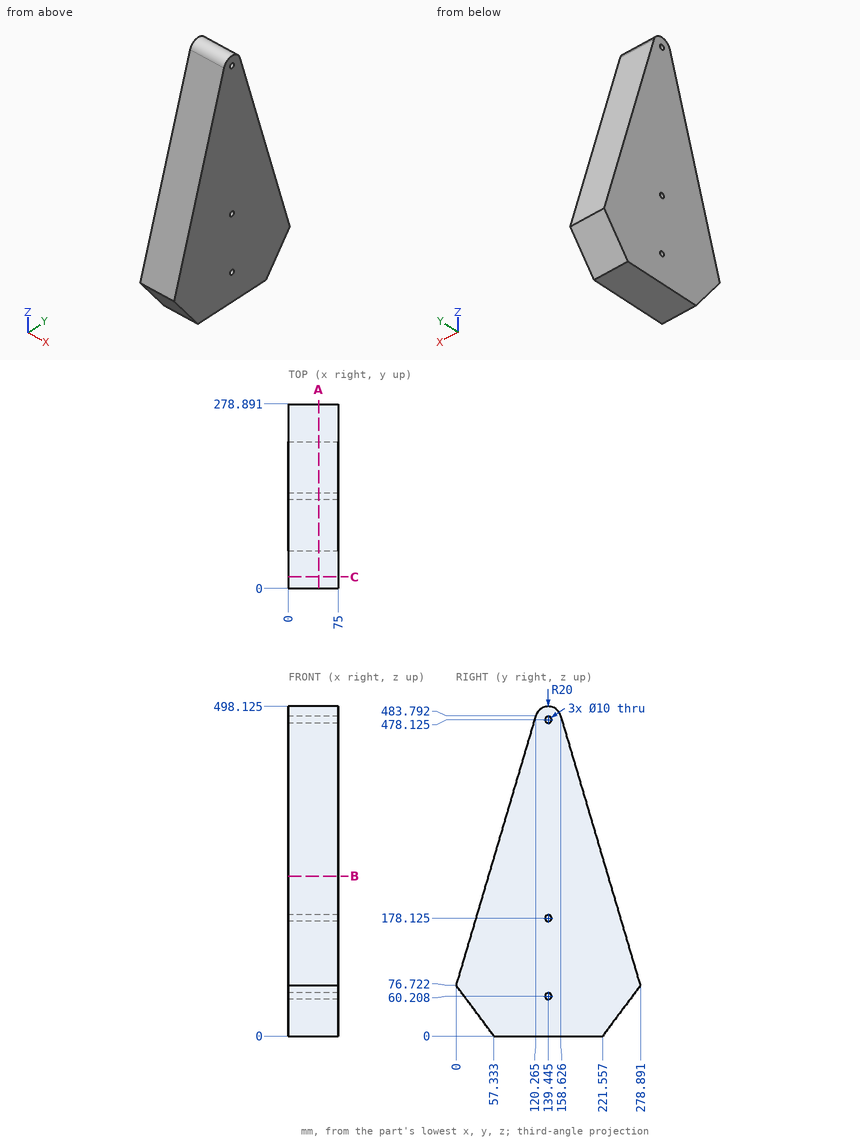
Answer from the drawing. Dimensions are ordinates in mm from the lowest x, y and z of the part. Round coordinates to 2 decimals unless told otherwise and drop trailing zeros. Loops run counter-clockwise (first coordinate to the right, second up) from the corner with the lowest first, then second, coordinate; pieces in that order, holes last. Notation, with made-up numbers: M 41,56.25 L 98,56.25 A14 cw 98,82.25 Z; hole C -5,20.25 d7. An arc over 180 degrees is marked long. One line per question, with ' | ' between items. Start each with the question number.
(1) A cutting plane is placed at A-A on x = 45.5. Write down the section's boundary in (y, z) (1 decimal).
(2) A cutting plane is placed at B-B on z = 241.5. Write down the section's boundary in (x, y).
(3) Find the intervals of material crossed by line 1 (Y direction, x = 33, z = 445) (1 decimal); line 2 (Z direction, x = 39.5, y = 126.5); line 3 (Y direction, x = 16, z = 472.5), in increasing order.
(4) A cutting plane is placed at C-C on y = 17.5. Write down the section's boundary in (x, z) (1 decimal).
(5) Flat-ended cylindrical pins translate along their axes: pin 1 Ø2 at (x, z) = (21.5, 366.5) entering from -Y; pin 2 Ø2 at (y, z) = (71, 207) entering from -X; pin 3 Ø1 at (x, z) = (60.5, 431) entering from -Y; pin 4 Ø10 at (x, z) = (14, 283) entering from +Y (1 decimal). Find the tip coordinate at first contact, or state that the pin passes through.
Geometry check:
1) outline: M 0,76.7 L 57.3,0 L 221.6,0 L 278.9,76.7 L 158.6,483.8 A20 ccw 120.3,483.8 Z; hole C 139.4,60.2 d10; hole C 139.4,178.1 d10; hole C 139.4,478.1 d10
2) outline: M 0,48.68 L 75,48.68 L 75,230.21 L 0,230.21 Z
3) line 1: y = 108.8 to 170.1 | line 2: z = 0 to 493.37 | line 3: y = 116.93 to 161.96
4) outline: M 0,53.3 L 75,53.3 L 75,136 L 0,136 Z
5) pin 1: stops at y = 85.32 | pin 2: stops at x = 0 | pin 3: stops at y = 104.52 | pin 4: stops at y = 219.4
